The drawing under review shows one solid part. Ordinate dimensions are in mm from its lowest x, y, z. Coordinates: 2 decimals unless noted, no trailing zeros. Order: outer loops, then holes, each group sorted by start corner. A loop starts at its lowest first (then second) coordinate and runs counter-clockwise, first axis right, second up.
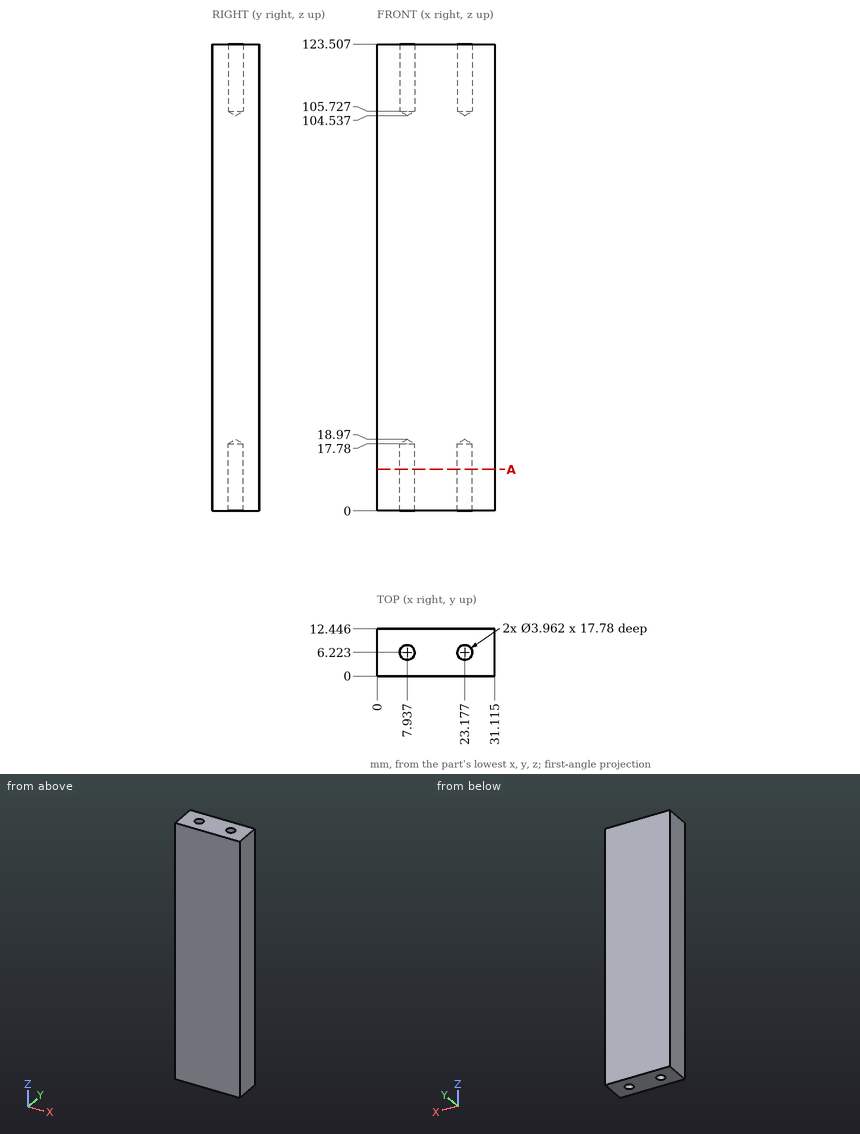
1. Insertion check: pin 1 (6.5 mm diameter, centred on x = 23.18, y = 6.22, fed in from +Z); pin 2 (2.5 mm diameter, centred on x = 7.94, y = 6.22, fed in from -Z). Each pin has a flat end and moves straight along its axis. Give the tip position at first contact, or say it passes through.
2. Add section A-A (z = 11). Give the boundary of the cut face in (x, y) (1 decimal).
3. To check wall thickness, follow line 1 (X direction, y = 7.75, z = 106) (1 decimal); line 2 (Y direction, x = 22.5, z = 6) (1 decimal). State the ranges of each line that lie inside material, in increasing order.
Solution:
1. pin 1: stops at z = 123.51
1. pin 2: stops at z = 18.22
2. outline: (0, 0) - (31.1, 0) - (31.1, 12.4) - (0, 12.4) - close; hole circle Ø4 at (7.9, 6.2); hole circle Ø4 at (23.2, 6.2)
3. line 1: x = 0 to 6.7, 9.2 to 21.9, 24.4 to 31.1
3. line 2: y = 0 to 4.4, 8.1 to 12.4
